Could you check a few things on this model? Use its own coordinates, in mm. Give positions to 0.01 mm unless a question says otherwise; leave off trailing zeros. Loops run counter-clockwise (first coordinate to the right, second up) from the corner with the lowest first, then second, coordinate; pieces in that order, holes last.
1. I need wall thicknesses on line 1 along Y through (x, z) = (57.5, 0.8); line 2 along X through (y, z) = (6, 0.2). Which ranges of each line are inside material? Lowest first, please.
2. For P1, Ø8, axis at x = -30, y = 23, coming from the -Z side, with a flat end and sliding along its axis, tell me the tip position at first contact or that it passes through.
3. Imagine slicing it at B-B (x = -57.5). List the corners of the cut face in (y, z) for me.
4. Imagine slicing it at A-A (y = 5). List the corners of the cut face in (x, z) for me.
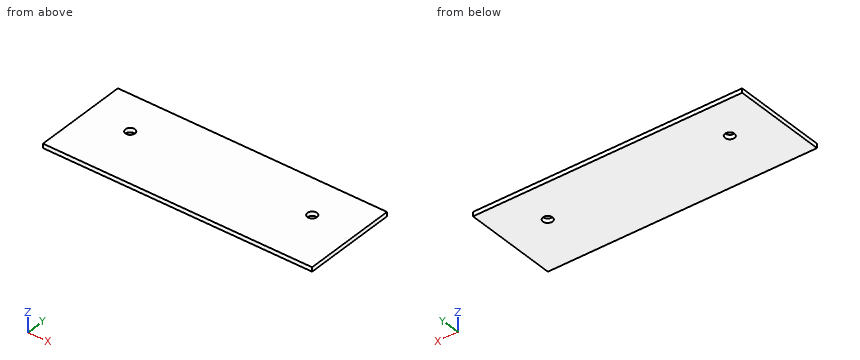
Solid Edge part; units mm, degrees
sketch "Sketch1" plane through (0, 0, 0) normal (0, 0, 1) x (1, 0, 0)
  line L0 (-85, -30) -> (85, -30)
  line L1 (85, -30) -> (85, 30)
  line L2 (85, 30) -> (-85, 30)
  line L3 (-85, 30) -> (-85, -30)
  dimension "D1" = 85
  dimension "D2" = 85
extrude "Protrusion1" add sketch "Sketch1" along normal blind 2.72
sketch "Sketch2" plane through (0, 0, 2.72) normal (0, 0, 1) x (1, 0, 0)
  circle A0 centre (-57.5, 5) radius 3
  circle A1 centre (57.5, 5) radius 3
  dimension "D1" = 57.5
extrude "Cutout1" cut sketch "Sketch2" against normal through all
properties material "Nylon, allgemein"
Derived:
1. line 1: y = -30 to 2, 8 to 30
1. line 2: x = -85 to -60.33, -54.67 to 54.67, 60.33 to 85
2. P1: stops at z = 0
3. outline: (-30, 0) - (2, 0) - (2, 2.72) - (-30, 2.72) - close; (8, 0) - (30, 0) - (30, 2.72) - (8, 2.72) - close
4. outline: (-85, 0) - (-60.5, 0) - (-60.5, 2.72) - (-85, 2.72) - close; (-54.5, 0) - (54.5, 0) - (54.5, 2.72) - (-54.5, 2.72) - close; (60.5, 0) - (85, 0) - (85, 2.72) - (60.5, 2.72) - close
